Read the model definition and answer for the solid it produces. Units are mm, in the model's axes. A direction names the side the tool comes from. Coordinates: 2 decimals unless noted, no trailing zeros. Order: outer loops, then holes, each group sorted by start corner. A loop starts at its lowest first (then second) coordinate and runs counter-clockwise, first axis right, second up. Notation, with made-up numbers: (-36.5, 0.25) - (-29.5, 0.25) arc R25 cw to (-29.5, 32.25) - close; hole circle Ø3 at (86, 37). An arc over 180 degrees is marked (long way). Use one line per item in the form item = value.
```python
from build123d import *

# Parameters (mm, degrees)
F0_W      = 304.8
F0_H      = 8
F1_DEPTH  = 8
F2_DEPTH  = 25.4
F3_W      = 19.05
F3_H      = 25.4
F4_DEPTH  = 2.5
F6_W      = 8
F6_H      = 8
F7_DEPTH  = 25
F9_DEPTH  = 8
F12_DEPTH = 609.6
F13_DEPTH = 609.6
F15_DEPTH = 2.5
F17_DEPTH = 2.5
F18_R     = 2
F19_DEPTH = 13


with BuildPart() as f1:
    # F0 (on Top) → F1 (new body)
    with BuildSketch(Plane.XY):
        with Locations((0, 51)):
            Rectangle(F0_W, F0_H)
    extrude(amount=F1_DEPTH)



with BuildPart() as f1b:
    # F0 (on Top) → F1, piece 2 (new body)
    with BuildSketch(Plane.XY):
        with Locations((0, -51)):
            Rectangle(F0_W, F0_H)
    extrude(amount=F1_DEPTH)


with BuildPart() as f1_1:
    add(f1.part)

    add(f1b.part)  # F2 merges F1b
    # F0 (on Top) → F2 (join)
    with BuildSketch(Plane.XY):
        Polygon((-152.4, 47), (-152.4, 55), (-154.9, 55), (-154.9, -55), (-152.4, -55), (-152.4, -47), align=None)
        Polygon((154.9, 55), (152.4, 55), (152.4, 47), (152.4, -47), (152.4, -55), (154.9, -55), align=None)
    extrude(amount=F2_DEPTH)

    # F3 (on face) → F4 (join)
    with BuildSketch(Plane.XZ.offset(55)):
        with Locations((-145.375, 12.7)):
            Rectangle(F3_W, F3_H)
        with Locations((145.375, 12.7)):
            Rectangle(F3_W, F3_H)
    extrude(amount=F4_DEPTH)

    # F5: F1 across plane


with BuildPart() as f1_2:
    add(f1_1.part)
    add(f1_1.part.mirror(Plane.XZ))

    # F6 (on face) → F7 (join)
    with BuildSketch(Plane.XY.offset(8)):
        with Locations((148.4, -51)):
            Rectangle(F6_W, F6_H)
    extrude(amount=F7_DEPTH)

    # F8 (on face) → F9 (cut)
    with BuildSketch(Plane(origin=(0, -47, 0), x_dir=(-1, 0, 0), z_dir=(0, 1, 0))):
        Polygon((-152.4, 9.9575875458), (-144.4, 8), (-144.4, 33), (-152.4, 33), (-152.4, 25.4), align=None)
    extrude(amount=-F9_DEPTH, mode=Mode.SUBTRACT)

    # F10: F1 across plane


with BuildPart() as f1_3:
    add(f1_2.part)
    add(f1_2.part.mirror(Plane.XZ))

    # F11: F1 across plane


with BuildPart() as f1_4:
    add(f1_3.part)
    add(f1_3.part.mirror(Plane.YZ))

    # F12 (add): faces of the model
    f12_faces = [f1_4.faces().sort_by_distance(p)[0] for p in [
        (148.4, 51, 8.9787937729),
        (148.4, -51, 8.9787937729),
    ]]
    extrude(f12_faces, amount=F12_DEPTH)

    # F13 (add): faces of the model
    f13_faces = [f1_4.faces().sort_by_distance(p)[0] for p in [
        (-148.4, 51, 8.9787937729),
        (-148.4, -51, 8.9787937729),
    ]]
    extrude(f13_faces, amount=F13_DEPTH)

    # F14 (on face) → F15 (join)
    with BuildSketch(Plane(origin=(0, 55, 0), x_dir=(-1, 0, 0), z_dir=(0, 1, 0))):
        Polygon((7.506680038, 602.087713304), (-7.506680038, 602.087713304), (-12.5, 581.6816988801), (12.5, 581.6816988801), align=None)
    extrude(amount=F15_DEPTH)

    # F16 (on face) → F17 (join)
    with BuildSketch(Plane.XZ.offset(-47)):
        Polygon((7.506680038, 602.087713304), (-7.506680038, 602.087713304), (-12.5, 581.6816988801), (12.5, 581.6816988801), align=None)
    extrude(amount=F17_DEPTH)

    # F18 (on face) → F19 (cut, through all)
    with BuildSketch(Plane(origin=(0, 57.5, 0), x_dir=(-1, 0, 0), z_dir=(0, 1, 0))):
        with Locations((0, 592.087713304)):
            Circle(F18_R)
    extrude(amount=-F19_DEPTH, mode=Mode.SUBTRACT)

    # F20: F1 across plane


with BuildPart() as f1_5:
    add(f1_4.part)
    add(f1_4.part.mirror(Plane.XZ))


solid = f1_5.part
```
(1) The mould has two halves that part along X. Classify faces 3 (the flat face through (152.4, 1, 13)), 4 (the flat face through (-77, -55, 300)): +X half, -X half, draft (parallel to the pull), parting line (faces both ways), or undercut.
Answer list:
face_3 = undercut
face_4 = draft
(2) Straight lines are drawn through the part: L1, parallel to Z at x = 0, y = -46.25; L2, parallel to X at y = 50.5, z = 290. For each, find the intervals that lie inside material, in ascending order.
Answer list:
L1 = 581.68 to 590.09, 594.09 to 602.09
L2 = -83.87 to -75.4, 75.4 to 83.87
(3) Section B-B, the plane x = -119.5 is taken. Write down the section's boundary in (y, z), then the cut area to 3 significant figures.
Answer list:
outline = (-55, 0) - (-47, 0) - (-47, 8) - (-55, 8) - close; (-55, 109.76) - (-47, 109.76) - (-47, 144.41) - (-55, 144.41) - close; (47, 0) - (55, 0) - (55, 8) - (47, 8) - close; (47, 109.76) - (55, 109.76) - (55, 144.41) - (47, 144.41) - close
area = 682 mm2
(4) Section A-A, the plane y = -13.5 is taken. Write down the section's boundary in (x, z).
Answer list:
outline = (-154.9, 0) - (-152.4, 0) - (-152.4, 25.4) - (-154.9, 25.4) - close; (152.4, 0) - (154.9, 0) - (154.9, 25.4) - (152.4, 25.4) - close
(5) Given pin 1 Ø12 at (y, z) = (-45, 150) entering from +X; pin 2 Ø2 at (x, y) = (3, 45.5) entering from -Z, each flat-ended and moving along its own axis, determine where each tip first touches the part or whether it passes through.
Answer list:
pin_1 = 119.52
pin_2 = 581.68
(6) Which of the six approach directions +Z, -Z, +X, -X, +Y, -Y give full straight-line access (tool end or side, diameter ignored) to faces 1 (the flat face through (145, 57.5, 13)), 2 (the flat face through (-0.2, 44.5, 589.8))?
Answer list:
face_1 = +Z, -Z, +X, -X, +Y
face_2 = +Z, -Z, +X, -X
(7) Section C-C, the plane z = 232 is taken. Write down the section's boundary in (x, y).
Answer list:
outline = (-98.07, -55) - (-89.59, -55) - (-89.59, -47) - (-98.07, -47) - close; (-98.07, 47) - (-89.59, 47) - (-89.59, 55) - (-98.07, 55) - close; (89.59, -55) - (98.07, -55) - (98.07, -47) - (89.59, -47) - close; (89.59, 47) - (98.07, 47) - (98.07, 55) - (89.59, 55) - close
